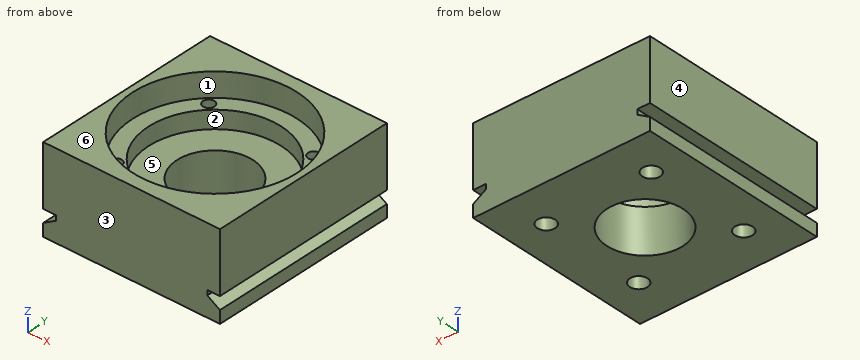
from build123d import *

# Parameters (mm, degrees)
F1_DEPTH = 75
F5_R     = 7
F6_DEPTH = 12
F4_R     = 4.5
F7_DEPTH = 37
F9_DEPTH = 150


with BuildPart() as f1:
    # F0 (on Front) → F1 (new body, symmetric)
    with BuildSketch(Plane.XZ):
        Polygon((-70, 0), (0, 0), (70, 0), (70, 68), (-70, 68), align=None)
    extrude(amount=F1_DEPTH, both=True)

    # F2 (on Front) → F3 (revolve, cut)
    with BuildSketch(Plane.XZ):
        Polygon((0, 68), (0, 0), (30, 0), (30, 35), (52.5, 35), (52.5, 49), (65, 49), (65, 68), align=None)
    revolve(axis=Axis((0, 0, 34), (0, 0, 1)), mode=Mode.SUBTRACT)

    # F5 (on face) → F6 (cut)
    with BuildSketch(Plane(origin=(0, 0, 0), x_dir=(1, 0, 0), z_dir=(0, 0, -1))):
        with Locations((41.577879, 41.577879)):
            Circle(F5_R)
        with Locations((41.577879, -41.577879)):
            Circle(F5_R)
        with Locations((-41.577879, -41.577879)):
            Circle(F5_R)
        with Locations((-41.577879, 41.577879)):
            Circle(F5_R)
    extrude(amount=-F6_DEPTH, mode=Mode.SUBTRACT)

    # F4 (on face) → F7 (cut, symmetric)
    with BuildSketch(Plane.XY.offset(35)):
        with Locations((41.577879, 41.577879)):
            Circle(F4_R)
        with Locations((41.577879, -41.577879)):
            Circle(F4_R)
        with Locations((-41.577879, -41.577879)):
            Circle(F4_R)
        with Locations((-41.577879, 41.577879)):
            Circle(F4_R)
    extrude(amount=F7_DEPTH, both=True, mode=Mode.SUBTRACT)

    # F8 (on face) → F9 (cut)
    with BuildSketch(Plane.XZ.offset(75)):
        Polygon((60, 16), (70, 10), (70, 20), (60, 20), align=None)
        Polygon((-60, 16), (-60, 20), (-70, 20), (-70, 10), align=None)
    extrude(amount=-F9_DEPTH, mode=Mode.SUBTRACT)


solid = f1.part
For this review, take the finished solid that the model builds, in its own axes (mm). Face numbers are marked on the shaded views. A direction names the side the tool comes from. Round coordinates to 2 decimals unless told otherwise and drop trailing zeros. Write each loop counter-clockwise with the first axis right and the second up, starting at its lowest first coordinate (ties: lowest second). Pieces come first, ordered by that corner, then holes. Notation, with made-up numbers: (-24.75, -34) -> (-7.75, -34) arc R19 cw to (-7.75, -17) -> close; hole circle Ø6 at (84, 42). An arc over 180 degrees is marked (long way). Use CSV: the item, a comma, the result in double quotes.
(1) Consider section C-C, the plane z = 44. Give the boundary of the cut face in (x, y).
Computed values:
outline,"(-70, -75) -> (70, -75) -> (70, 75) -> (-70, 75) -> close; hole circle Ø105 at (0, 0); hole circle Ø9 at (-41.58, -41.58); hole circle Ø9 at (-41.58, 41.58); hole circle Ø9 at (41.58, -41.58); hole circle Ø9 at (41.58, 41.58)"
(2) Consider section A-A, the plane x = 0. Give the boundary of the cut face in (y, z), plus the area to 3 significant figures.
Computed values:
outline,"(-75, 0) -> (-30, 0) -> (-30, 35) -> (-52.5, 35) -> (-52.5, 49) -> (-65, 49) -> (-65, 68) -> (-75, 68) -> close; (30, 0) -> (75, 0) -> (75, 68) -> (65, 68) -> (65, 49) -> (52.5, 49) -> (52.5, 35) -> (30, 35) -> close"
area,"4,160 mm²"
(3) Consider section B-B, the plane y = 0. Give the boundary of the cut face in (x, z).
Computed values:
outline,"(-70, 0) -> (-30, 0) -> (-30, 35) -> (-52.5, 35) -> (-52.5, 49) -> (-65, 49) -> (-65, 68) -> (-70, 68) -> (-70, 20) -> (-60, 20) -> (-60, 16) -> (-70, 10) -> close; (30, 0) -> (70, 0) -> (70, 10) -> (60, 16) -> (60, 20) -> (70, 20) -> (70, 68) -> (65, 68) -> (65, 49) -> (52.5, 49) -> (52.5, 35) -> (30, 35) -> close"
(4) For the marked faces 5 and 6, list the 3-axis set-ups (+Z, -Z, +X, -X, +Y, -Y) from which the entire face can be reached by the end or side of a thin tool; tool diameter is ignored.
Computed values:
face 5,"+Z"
face 6,"+Z, +X, -X, +Y, -Y"
(5) Clearance check with flat-ended pins moving along their axes: P1, Ø4, axis at x = -39, y = -42.5, coming from the -Z side; P2, Ø11, axis at x = 41.58, y = 41.58, coming from the +Z side. State where each tip first meets the part, or that it passes through.
Computed values:
P1,"z = 12"
P2,"z = 49"
(6) Consider section D-D, the plane y = 20.5. Give the boundary of the cut face in (x, z), plus the area to 3 significant figures.
Computed values:
outline,"(-70, 0) -> (-21.9, 0) -> (-21.9, 35) -> (-48.33, 35) -> (-48.33, 49) -> (-61.68, 49) -> (-61.68, 68) -> (-70, 68) -> (-70, 20) -> (-60, 20) -> (-60, 16) -> (-70, 10) -> close; (21.9, 0) -> (70, 0) -> (70, 10) -> (60, 16) -> (60, 20) -> (70, 20) -> (70, 68) -> (61.68, 68) -> (61.68, 49) -> (48.33, 49) -> (48.33, 35) -> (21.9, 35) -> close"
area,"4,150 mm²"
(7) To check wall thickness, follow L1, parallel to X at y = -41.5, z = 19.5; L2, parallel to X at y = -45, z = 21; L3, parallel to Y at x = 40, z = 22. State the ranges of each line that lie inside material, in increasing order. Write a range as [from, to].
Computed values:
L1,"[-60, -46.08], [-37.08, 37.08], [46.08, 60]"
L2,"[-70, -44.5], [-38.66, 38.66], [44.5, 70]"
L3,"[-75, -45.79], [-37.36, 37.36], [45.79, 75]"
(8) Draft analysis for pull direction X (two halves, no side actions). For the marked faces 1, 2, 3 and 4, state which applies: +X half, -X half, draft (parallel to the pull), parting line (faces both ways), or undercut.
Computed values:
face 1,"undercut"
face 2,"undercut"
face 3,"draft"
face 4,"-X half"
